```python
from build123d import *

# Parameters (mm, degrees)
F0_R     = 27.5
F0_R_2   = 26.5
F1_DEPTH = 65
F0_R_3   = 2.15
F0_R_4   = 14.25
F0_R_5   = 1.65
F2_DEPTH = 3
F3_DEPTH = 2


with BuildPart() as f1:
    # F0 (on Top) → F1 (new body)
    with BuildSketch(Plane.XY):
        Circle(F0_R)
        Circle(F0_R_2, mode=Mode.SUBTRACT)
    extrude(amount=F1_DEPTH)

    # F0 (on Top) → F2 (join)
    with BuildSketch(Plane.XY):
        Circle(F0_R)
        Circle(F0_R_2, mode=Mode.SUBTRACT)
        Circle(F0_R_2)
        with Locations((0, -19.25)):
            Circle(F0_R_3, mode=Mode.SUBTRACT)
        with Locations((-19.25, 0)):
            Circle(F0_R_3, mode=Mode.SUBTRACT)
        Circle(F0_R_4, mode=Mode.SUBTRACT)
        with Locations((19.25, 0)):
            Circle(F0_R_3, mode=Mode.SUBTRACT)
        with Locations((0, 19.25)):
            Circle(F0_R_3, mode=Mode.SUBTRACT)
        Circle(F0_R_4)
        with Locations((5.678908, -10)):
            Circle(F0_R_5, mode=Mode.SUBTRACT)
        with Locations((-9, 0)):
            Circle(F0_R_5, mode=Mode.SUBTRACT)
        with Locations((-5.678908, 10)):
            Circle(F0_R_5, mode=Mode.SUBTRACT)
        with Locations((9, 0)):
            Circle(F0_R_5, mode=Mode.SUBTRACT)
    extrude(amount=-F2_DEPTH)

    # F0 (on Top) → F3 (join)
    with BuildSketch(Plane.XY):
        Circle(F0_R_2)
        with Locations((0, -19.25)):
            Circle(F0_R_3, mode=Mode.SUBTRACT)
        with Locations((-19.25, 0)):
            Circle(F0_R_3, mode=Mode.SUBTRACT)
        Circle(F0_R_4, mode=Mode.SUBTRACT)
        with Locations((19.25, 0)):
            Circle(F0_R_3, mode=Mode.SUBTRACT)
        with Locations((0, 19.25)):
            Circle(F0_R_3, mode=Mode.SUBTRACT)
    extrude(amount=F3_DEPTH)


solid = f1.part
```
For this review, take the finished solid that the model builds, in its own axes (mm). A direction names the side the tool comes from. Give positions to 0.01 mm unless a question says otherwise; leave off trailing zeros. Write each loop counter-clockwise with the first axis right and the second up, starting at its lowest first coordinate (ties: lowest second). Pieces come first, ordered by that corner, then holes. Notation, with made-up numbers: M 54,25 L 83,25 A27 ccw 83,50 Z; hole C 61.5,0 d8. An arc over 180 degrees is marked long. One line per item, written item: value.
1) Take a section at A-A, the plane y = 0. Write out the cut boundary in (x, z).
Results are:
outline: M -27.5,-3 L -21.4,-3 L -21.4,2 L -26.5,2 L -26.5,65 L -27.5,65 Z; M -17.1,-3 L -10.65,-3 L -10.65,0 L -14.25,0 L -14.25,2 L -17.1,2 Z; M -7.35,-3 L 7.35,-3 L 7.35,0 L -7.35,0 Z; M 10.65,-3 L 17.1,-3 L 17.1,2 L 14.25,2 L 14.25,0 L 10.65,0 Z; M 21.4,-3 L 27.5,-3 L 27.5,65 L 26.5,65 L 26.5,2 L 21.4,2 Z
2) Take a section at C-C, the plane z = 3. Write out the cut boundary in (x, y), then the cut area to 3 significant figures.
Results are:
outline: C 0,0 d55; hole C 0,0 d53
area: 170 mm²
3) Take a section at D-D, the plane y = 19.25. Write out the cut boundary in (x, z), then the cut area to 3 significant figures.
Results are:
outline: M -19.64,-3 L -2.15,-3 L -2.15,2 L -18.21,2 L -18.21,65 L -19.64,65 Z; M 2.15,-3 L 19.64,-3 L 19.64,65 L 18.21,65 L 18.21,2 L 2.15,2 Z
area: 355 mm²
4) Take a section at B-B, the plane x = -6. Write out the cut boundary in (y, z).
Results are:
outline: M -26.84,-3 L 8.38,-3 L 8.38,0 L -12.93,0 L -12.93,2 L -25.81,2 L -25.81,65 L -26.84,65 Z; M 11.62,-3 L 26.84,-3 L 26.84,65 L 25.81,65 L 25.81,2 L 12.93,2 L 12.93,0 L 11.62,0 Z
5) The part is to be moulded in two halves that separate along X. For faces 3 (the cylindrical face through (-5.961, -26.846, 31.476)), 4 (the cylindrical face through (-0.47, 17.15, -0.54)), 5 (the flat face through (0, 0, -3)), say which applies: +X half, -X half, draft (parallel to the pull), parting line (faces both ways), or undercut.
Results are:
face 3: parting line
face 4: undercut
face 5: draft
6) For faces 1 (the cylindrical face through (-4.155, 9.368, -1.479)), 2 (the cylindrical face through (13.163, -5.458, 0.986)), list the 3-axis set-ups (+Z, -Z, +X, -X, +Y, -Y) from which the entire face can be reached by the end or side of a thin tool; tool diameter is ignored.
Results are:
face 1: +Z, -Z
face 2: +Z
7) For P1, Ø4, axis at x = -15.5, z = 30.5, coming from the +Y side; P2, Ø1.5, axis at y = -6, z = 31.5, coming from the +X side; P3, Ø2.5, axis at x = 19.25, y = 0, coming from the -Z side; P4, Ø16, axis at x = 13, y = 7.5, coming from the +Z side, all flat-tipped, find the tip position at first contact; note any pin that passes through.
Results are:
P1: stops at y = 23.96
P2: stops at x = 26.99
P3: passes through
P4: stops at z = 2
8) For line 1 (X direction, y = -1, z = 36); line 2 (Z direction, x = 2, y = -0.5); line 3 (Y direction, x = 9, z = 50), list the stretches that pass through material, from the lowest coordinate up. Write a range as from..to.
Results are:
line 1: x = -27.48..-26.48, 26.48..27.48
line 2: z = -3..0
line 3: y = -25.99..-24.92, 24.92..25.99
